Work out the finished part from the listing and answer in its coordinate system (mm). A direction names the side the tool comes from. Give positions to 0.01 mm unless a question says otherwise; leave off trailing zeros. Order: outer loops, then holes, each group sorted by start corner. A loop starts at its lowest first (then second) coordinate and runs counter-clockwise, first axis right, second up. Notation, with made-up numbers: (-26.75, 28) -> (25.25, 28) arc R13 cw to (25.25, 37) -> close; hole circle Ø11 at (66.5, -6.75). An arc over 180 degrees is marked (long way). Answer as CSV lines item,"result". Start each with the question number.
1. Find the intervals of material crossed by L1, parallel to Z at x = -2.5, y = 4; L2, parallel to Z at x = 5.25, y = 8.25; L3, parallel to Y at x = -7, z = -53, in increasing order.
2. A cutting plane is placed at A-A (z = 14.5). Give the vertices of the cut face in (x, y), then the cut area to 3 significant figures.
3. For faces 1 (the cylindrical face through (-1.172, -8.923, -6.902)), 2 (the flat face through (0, 0, 45)), 3 (the conical face through (5.154, -1.623, -127.185)), determine the directions among +Z, -Z, +X, -X, +Y, -Y from which every point of the face is accessible in a straight line to the end or side of a thin tool.
4. Flat-ended cylindrical pins translate along their axes: pin 1 (3 mm diameter, centred on x = 7.5, y = 7, fed in from +Z); pin 2 (9 mm diameter, centred on x = 3.5, y = 2.5, fed in from +Z); pin 3 (4 mm diameter, centred on y = 1.5, z = -46, fed in from -X); pin 4 (8 mm diameter, centred on x = -5.5, z = -51.5, fed in from -Y). Find the tip coordinate at first contact, or state that the pin passes through.
5. A cutting plane is placed at B-B (z = -85.5). Give the vertices of the cut face in (x, y) (3 decimals).
from build123d import *


with BuildPart() as f1:
    # F0 (on Front) → F1 (revolve)
    with BuildSketch(Plane.XZ):
        with BuildLine():
            Line((0, 45), (0, -150))
            Line((0, -150), (5, -150))
            Line((5, -150), (5.795, -105))
            Line((5.795, -105), (5.795, -55.255))
            Line((5.795, -55.255), (7.85, -53.2))
            Line((7.85, -53.2), (7.85, -24.316154))
            ThreePointArc((7.85, -24.316154), (8.420641, -19.572738), (10.1, -15.1))
            Line((10.1, -15.1), (9, -14))
            Line((9, -14), (9, 0))
            Line((9, 0), (3.75, 0))
            Line((3.75, 0), (3.75, 45))
            Line((3.75, 45), (0, 45))
        make_face()
    revolve(axis=Axis((0, 0, -52.5), (0, 0, -1)))


solid = f1.part
Answer sheet:
1,L1,"z = -150 to 0"
1,L2,"z = -15.75 to -14.78"
1,L3,"y = -3.55 to 3.55"
2,outline,"circle Ø7.5 at (0, 0)"
2,area,"44.2 mm^2"
3,face 1,"+Z"
3,face 2,"+Z, +X, -X, +Y, -Y"
3,face 3,"-Z"
4,pin 1,"stops at z = 0"
4,pin 2,"stops at z = 45"
4,pin 3,"stops at x = -7.85"
4,pin 4,"stops at y = -7.71"
5,outline,"circle Ø11.59 at (0, 0)"
